Autodesk Inventor part; units mm, degrees
ref_plane "YZ Plane" through (0, 0, 0) normal (1, 0, 0) x (0, 1, 0)
ref_plane "XZ Plane" through (0, 0, 0) normal (0, 1, 0) x (-1, 0, 0)
ref_plane "XY Plane" through (0, 0, 0) normal (0, 0, 1) x (1, 0, 0)
sketch "Sketch1" plane through (0, 0, 0) normal (0, 0, 1) x (1, 0, 0)
  line L0 (-10, 5.5) -> (-0.289, 5.5)
  line L1 (10, 5) -> (10, -5.5)
  line L2 (10, -5.5) -> (-10, -5.5)
  line L3 (-10, -5.5) -> (-10, 5.5)
  line L4 (-0.289, 5.5) -> (0.4244, 5)
  line L5 (0.4244, 5) -> (10, 5)
  line L6 (-10, 5.5) -> (10, -5.5) construction
  circle A0 centre (4.75, -3.25) radius 1.25
  line L7 (0, -5.5) -> (0, 3.5475) construction
  circle A1 centre (-4.75, -3.25) radius 1.25
  point P0 (0, 0)
  point P1 (0, 0)
  point P2 (0, 0)
  dimension "d3" = 20
  dimension "d4" = 11
  dimension "d5" = 10.5
  dimension "d6" = 0.7134
  dimension "d7" = 2.5
  dimension "d8" = 2.25
  dimension "d9" = 5.25
extrude "Extrusion1" add sketch "Sketch1" along normal blind 6
sketch "Sketch2" plane through (-10, -5.5, 0) normal (0, -1, 0) x (1, 0, 0)
  line L0 (1.65, 4.5) -> (2.15, 4.5)
  line L1 (2.15, 4.5) -> (2.15, 1.5)
  line L2 (2.15, 1.5) -> (1.65, 1.5)
  line L3 (1.65, 1.5) -> (1.65, 4.5)
  line L4 (10.65, 4.5) -> (11.15, 4.5)
  line L5 (11.15, 4.5) -> (11.15, 1.5)
  line L6 (11.15, 1.5) -> (10.65, 1.5)
  line L7 (10.65, 1.5) -> (10.65, 4.5)
  line L8 (17.85, 4.5) -> (18.35, 4.5)
  line L9 (18.35, 4.5) -> (18.35, 1.5)
  line L10 (18.35, 1.5) -> (17.85, 1.5)
  line L11 (17.85, 1.5) -> (17.85, 4.5)
  line L12 (0, 0) -> (0, 6)
  line L13 (0, 0) -> (20, 0)
  line L14 (0, 6) -> (20, 6)
  point P0 (10, 0)
  dimension "d12" = 3
  dimension "d13" = 3
  dimension "d14" = 3
  dimension "d15" = 0.5
  dimension "d16" = 0.5
  dimension "d17" = 0.5
  dimension "d18" = 1.65
  dimension "d19" = 8.5
  dimension "d20" = 6.7
  dimension "d21" = 6
  dimension "d22" = 1.5
extrude "Extrusion2" add sketch "Sketch2" along normal blind 4
sketch "Sketch3" plane through (8.35, -5.5, 4.5) normal (1, 0, 0) x (0, 0, -1)
  circle A0 centre (1.5, -2.5) radius 0.5
  line L0 (3, -4) -> (0, -4)
  line L1 (3, 0) -> (3, -4)
  line L2 (0, 0) -> (0, -4)
  point P0 (4.5, 5.5)
  dimension "d25" = 1
  dimension "d26" = 1.5
  dimension "d27" = 3
  dimension "d28" = 1.5
extrude "Extrusion3" cut sketch "Sketch3" against normal through all
chamfer "Chamfer1" distance 0.4 angle 45 6 edges at (8.1, -9.5, 4.5) (8.1, -9.5, 1.5) (0.9, -9.5, 1.5) (0.9, -9.5, 4.5) (-8.1, -9.5, 4.5) (-8.1, -9.5, 1.5)
fillet "Fillet1" radius 1 4 edges at (10, 5, 3) (10, -5.5, 3) (-10, -5.5, 3) (-10, 5.5, 3)
equation "\"d13\" = d12"
equation "\"d14\" = d13"
equation "\"d22\" = -0.5 * d12 + 0.5 * d21"
equation "\"d28\" = 0.5 * d27"
properties part number "limitSwitch"
For this review, take the finished solid that the model builds, in its own axes (mm). A direction names the side the tool comes from. Coordinates: 2 decimals unless noted, no trailing zeros. Write each loop counter-clockwise with the first axis right and the second up, starting at its lowest first coordinate (ties: lowest second). Pieces come first, ordered by that corner, then holes. Notation, with made-up numbers: (5, 88) - (18, 88) arc R11 ccw to (18, 97) - close; hole circle Ø2 at (62, 45.25). An arc over 180 degrees is marked (long way). Answer in a Markdown table with one row per item. Add a question column.
Q1. Tool access review of faces 4 (the flat face through (-8.35, -7, 3)), 5 (the flat face through (8.35, -7, 3)), 6 (the flat face through (1.15, -7, 3)), 7 (the cylindrical face through (5.94, -3.63, 2.96)), 8 (the flat face through (5, 5, 3)): name each direction out of +Z, -Z, +X, -X, +Y, -Y from which nothing blocks a thin tool from reaching the whole face with its end or side.
Q2. For probe 1 along Y at (x, z) = (1.05, 3); probe 2 along Y at (x, z) = (-4.75, 4.2); probe 3 along X at (y, z) = (-4.25, 2.15), list the stretches that pass through material, from the lowest coordinate up.
Q3. We need section C-C, the plane y = -8. State the section outline as (x, z) points.
Q4. We need section B-B, the plane x = -4.75. State the section outline as (y, z) points.
Q5. We need section A-A, the plane y = -2.5. State the section outline as (x, z) points, and give its area (3 significant figures).
Q6. Draft analysis for pull direction Z (two halves, no side actions). For faces 1 (the flat face through (0, 0, 6)), 2 (the cylindrical face through (0.904, -8.488, 3.108)), 3 (the cylindrical face through (-9.699, 5.215, 3.042)), state which applies: +Z half, -Z half, draft (parallel to the pull), parting line (faces both ways), or undercut.
Q7. For P1, Ø2, axis at x = -4.75, y = -3.25, coming from the -Z side; P2, Ø0.6, axis at x = -8, y = -8, coming from the +Z side; P3, Ø1.5, axis at y = -8.5, z = 2.5, coming from the -X side; P4, Ø1.8, axis at x = 5, z = 2, coming from the +Y side, all flat-tipped, find the tip position at first contact; note any pin that passes through.
Q8. We need section D-D, the plane z = 1.1. State the section outline as (x, y) points, and give its area (3 significant figures).
Answer list:
| question | item | result |
|---|---|---|
| 1 | face 4 | +Z, -Z, -X, -Y |
| 1 | face 5 | +Z, -Z, +X, -Y |
| 1 | face 6 | +Z, -Z, -Y |
| 1 | face 7 | +Z, -Z |
| 1 | face 8 | +Z, -Z, +X, +Y |
| 2 | probe 1 | y = -9.5 to -8.5, -7.5 to 5 |
| 2 | probe 2 | y = -5.5 to -4.5, -2 to 5.5 |
| 2 | probe 3 | x = -10 to -5.5, -4 to 4, 5.5 to 10 |
| 3 | outline | (-8.35, 1.5) - (-7.85, 1.5) - (-7.85, 2.5) - (-8.35, 2.5) - close; (-8.35, 3.5) - (-7.85, 3.5) - (-7.85, 4.5) - (-8.35, 4.5) - close; (0.65, 1.5) - (1.15, 1.5) - (1.15, 2.5) - (0.65, 2.5) - close; (0.65, 3.5) - (1.15, 3.5) - (1.15, 4.5) - (0.65, 4.5) - close; (7.85, 1.5) - (8.35, 1.5) - (8.35, 2.5) - (7.85, 2.5) - close; (7.85, 3.5) - (8.35, 3.5) - (8.35, 4.5) - (7.85, 4.5) - close |
| 4 | outline | (-5.5, 0) - (-4.5, 0) - (-4.5, 6) - (-5.5, 6) - close; (-2, 0) - (5.5, 0) - (5.5, 6) - (-2, 6) - close |
| 5 | outline | (-10, 0) - (-5.75, 0) - (-5.75, 6) - (-10, 6) - close; (-3.75, 0) - (3.75, 0) - (3.75, 6) - (-3.75, 6) - close; (5.75, 0) - (10, 0) - (10, 6) - (5.75, 6) - close |
| 5 | area | 96.0 mm2 |
| 6 | face 1 | +Z half |
| 6 | face 2 | undercut |
| 6 | face 3 | draft |
| 7 | P1 | passes through |
| 7 | P2 | stops at z = 4.5 |
| 7 | P3 | stops at x = -8.35 |
| 7 | P4 | stops at y = 5 |
| 8 | outline | (-10, -4.5) arc R1 ccw to (-9, -5.5) - (9, -5.5) arc R1 ccw to (10, -4.5) - (10, 4) arc R1 ccw to (9, 5) - (0.42, 5) - (-0.29, 5.5) - (-9, 5.5) arc R1 ccw to (-10, 4.5) - close; hole circle Ø2.5 at (-4.75, -3.25); hole circle Ø2.5 at (4.75, -3.25) |
| 8 | area | 204 mm2 |
